Work out the finished part from the listing and answer in its coordinate system (mm). Face numbers are marked on the shaded views. Give positions to 0.01 mm unless a question says otherwise; leave off trailing zeros. Loops run counter-clockwise (first coordinate to the right, second up) from the corner with the lowest first, then second, coordinate; pieces in that order, holes last. Notation, with made-up numbers: M 57,-9 L 102,-9 A18 ccw 102,3 Z; hole C -21.5,20 d11. An arc over 180 degrees is marked long. Write item = value, one per line. Start each with the question number.
1. Section B-B on x = 0 is taken. Determine the outline of the cut face in (y, z) (3 decimals).
2. Section A-A on y = 0 is taken. Determine the outline of the cut face in (x, z) (3 decimals), plus the area to 3 significant figures.
3. Flat-ended cylindrical pins translate along their axes: pin 1 Ø8.5 at (x, y) = (-9.62, -5.56) entering from -Z; pin 2 Ø0.6 at (y, z) = (5, 1) entering from -X. Find the tip coordinate at first contact, or state that the pin passes through.
4. The mould has two halves that part along X. Classify the marked faces 1, 2 and 3: released by +X, released by -X, zero draft, split by the parting line, or undercut.
5. Consider L1, parallel to Y at x = 0, z = 1.8 (3 decimals); L2, parallel to X at y = 6.5, z = 1.6; L3, parallel to Y at x = -9, z = 3. Determine where each line is inside the solid, lowest interval first. Write a range as [from, to].
6. Section D-D on z = 0.9 is taken. Give the number of separate pieces and of enclosed holes in the cut face, plus the area to 3 significant figures.
7. Section C-C on x = 10.5 is taken. Determine the outline of the cut face in (y, z) (3 decimals), plus the area to 3 significant figures.
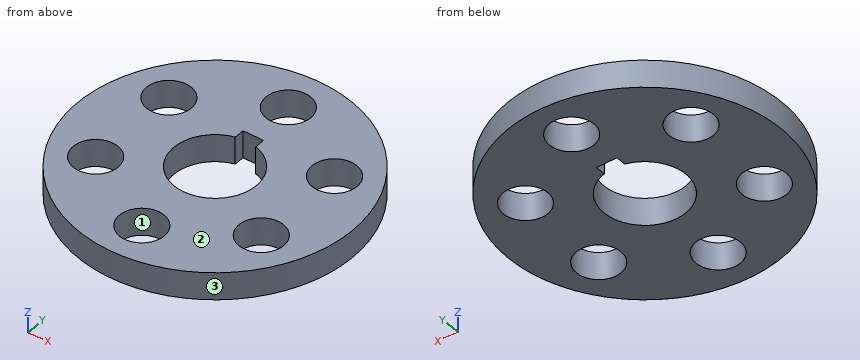
Autodesk Inventor part; units mm, degrees
ref_plane "YZ Plane" through (0, 0, 0) normal (1, 0, 0) x (0, 1, 0)
ref_plane "XZ Plane" through (0, 0, 0) normal (0, 1, 0) x (-1, 0, 0)
ref_plane "XY Plane" through (0, 0, 0) normal (0, 0, 1) x (1, 0, 0)
sketch "Sketch1" plane through (0, 0, 0) normal (0, 0, 1) x (1, 0, 0)
  arc A0 (-1.1906, 4.6113) -> (1.1906, 4.6113) centre (0, 0) ccw
  circle A1 centre (0, 0) radius 15.875
  line L0 (0, 4.7625) -> (0, 11.1125)
  circle A2 centre (0, 11.1125) radius 2.5908
  circle A3 centre (-9.6237, 5.5563) radius 2.5908
  circle A4 centre (-9.6237, -5.5562) radius 2.5908
  circle A5 centre (0, -11.1125) radius 2.5908
  circle A6 centre (9.6237, -5.5563) radius 2.5908
  circle A7 centre (9.6237, 5.5562) radius 2.5908
  line L1 (0, 0) -> (-1.1906, 0)
  line L2 (0, 0) -> (1.1906, 0)
  line L3 (1.1906, 0) -> (1.1906, 4.6113)
  line L4 (1.1906, 4.6113) -> (1.1906, 5.8019)
  line L5 (1.1906, 5.8019) -> (-1.1906, 5.8019)
  line L6 (-1.1906, 5.8019) -> (-1.1906, 4.6113)
  dimension "d0" = 9.525
  dimension "d1" = 31.75
  dimension "d2" = 6.35
  dimension "d3" = 5.1816
  dimension "d6" = 360
  dimension "d10" = 1.1906
  dimension "d11" = 1.1906
  dimension "d12" = 1.1906
extrude "Extrusion1" add sketch "Sketch1" along normal blind 3.175
properties part number "Hub for rachet" material "Steel"
Verdict:
q1.outline = M -15.875,0 L -13.703,0 L -13.703,3.175 L -15.875,3.175 Z; M -8.522,0 L -4.763,0 L -4.763,3.175 L -8.522,3.175 Z; M 5.802,0 L 8.522,0 L 8.522,3.175 L 5.802,3.175 Z; M 13.703,0 L 15.875,0 L 15.875,3.175 L 13.703,3.175 Z
q2.outline = M -15.875,0 L -4.763,0 L -4.763,3.175 L -15.875,3.175 Z; M 4.763,0 L 15.875,0 L 15.875,3.175 L 4.763,3.175 Z
q2.area = 70.6 mm2
q3.pin_1 = 0
q3.pin_2 = -15.16
q4.face_1 = undercut
q4.face_2 = zero draft
q4.face_3 = split by the parting line
q5.L1 = [-15.875, -13.703], [-8.522, -4.763], [5.802, 8.522], [13.703, 15.875]
q5.L2 = [-14.48, -12.04], [-7.21, 7.21], [12.04, 14.48]
q5.L3 = [-13.08, -8.07], [-3.04, 3.04], [8.07, 13.08]
q6.separate_pieces = 1
q6.enclosed_holes = 7
q6.area = 591 mm2
q7.outline = M -11.907,0 L -7.994,0 L -7.994,3.175 L -11.907,3.175 Z; M -3.118,0 L 3.118,0 L 3.118,3.175 L -3.118,3.175 Z; M 7.994,0 L 11.907,0 L 11.907,3.175 L 7.994,3.175 Z
q7.area = 44.6 mm2
